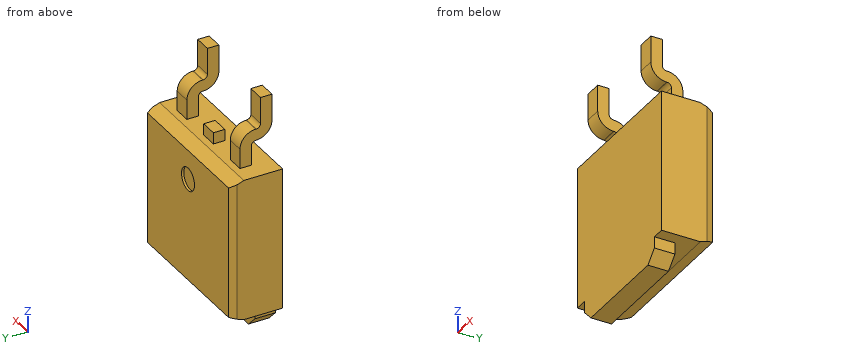
from build123d import *
from OCP.BRepFilletAPI import BRepFilletAPI_MakeChamfer

# Parameters (mm, degrees)
SKETCH1_W           = 6.5
SKETCH1_H           = 6.22
BOSS_EXTRUDE1_DEPTH = 2.3
SKETCH2_R           = 0.5
CUT_EXTRUDE1_DEPTH  = 0.1
SKETCH3_W           = 5.4
SKETCH3_H           = 0.9
BOSS_EXTRUDE2_DEPTH = 1
CHAMFER2_SIZE       = 0.5
SKETCH5_W           = 0.75
SKETCH5_H           = 0.5
SKETCH10_W          = 0.75
SKETCH10_H          = 0.5
BOSS_EXTRUDE3_DEPTH = 0.5
CHAMFER3_SIZE       = 0.6
CHAMFER3_SIZE2      = 0.218382141
CHAMFER4_SIZE       = 0.3
CHAMFER4_SIZE2      = 0.10919107


with BuildPart() as part:
    # Sketch1 → Boss-Extrude1 (new body)
    with BuildSketch(Plane(origin=(0, 0, 0), x_dir=(1, 0, 0), z_dir=(0, 1, 0))):
        with Locations((3.25, 3.11)):
            Rectangle(SKETCH1_W, SKETCH1_H)
    extrude(amount=BOSS_EXTRUDE1_DEPTH)

    # Sketch2 → Cut-Extrude1 (cut)
    with BuildSketch(Plane(origin=(0, 2.3, 0), x_dir=(1, 0, 0), z_dir=(0, 1, 0))):
        with Locations(Location((3.25, 1.5, 0), (0, 0, 270))):
            Circle(SKETCH2_R)
    extrude(amount=-CUT_EXTRUDE1_DEPTH, mode=Mode.SUBTRACT)

    # Sketch3 → Boss-Extrude2 (add)
    with BuildSketch(Plane(origin=(0, 0, -6.22), x_dir=(-1, 0, 0), z_dir=(0, 0, -1))):
        with Locations((-3.25, 0.45)):
            Rectangle(SKETCH3_W, SKETCH3_H)
    extrude(amount=BOSS_EXTRUDE2_DEPTH)

    # Chamfer2
    chamfer2_edges = [part.edges().sort_by_distance(p)[0] for p in [
        (5.95, 0.45, -7.22),
        (0.55, 0.45, -7.22),
    ]]
    chamfer(chamfer2_edges, length=CHAMFER2_SIZE)

    # Sweep2: sweep along a path in Sketch8
    with BuildLine(Plane(origin=(1.2, 0, 0), x_dir=(0, 0, -1), z_dir=(1, 0, 0))) as sweep2_path:
        Line((0, 1.15), (-0.860174932, 1.15))
        ThreePointArc((-0.860174932, 1.15), (-1.171301915, 1.021126984), (-1.300174932, 0.71))
        Line((-1.300174932, 0.71), (-1.300174932, 0.69))
        ThreePointArc((-1.300174932, 0.69), (-1.429047948, 0.378873016), (-1.740174932, 0.25))
        Line((-1.740174932, 0.25), (-2.900174932, 0.25))
    # Sketch5 → Sweep2 (sweep)
    with BuildSketch(Plane.XY):
        with Locations((1.2, 1.15)):
            Rectangle(SKETCH5_W, SKETCH5_H)
        with Locations((5.3, 1.15)):
            Rectangle(SKETCH5_W, SKETCH5_H)
    sweep(path=sweep2_path.line)

    # Sketch10 → Boss-Extrude3 (add)
    with BuildSketch(Plane.XY):
        with Locations((3.25, 1.15)):
            Rectangle(SKETCH10_W, SKETCH10_H)
    extrude(amount=BOSS_EXTRUDE3_DEPTH)

    # Chamfer3: one chamfer whose edges measure the first distance from different faces: ONE call of the kernel's chamfer builder (chamfer() names one face for all edges)
    chamfer3_edges_1 = [part.edges().sort_by_distance(p)[0] for p in [
        (3.25, 2.3, -6.22),
    ]]
    chamfer3_side_1 = [part.faces().sort_by_distance(p)[0] for p in [
        (3.25, 1.48716551, -6.22),
    ]]
    chamfer3_edges_2 = [part.edges().sort_by_distance(p)[0] for p in [
        (3.25, 2.3, 0),
    ]]
    chamfer3_side_2 = [part.faces().sort_by_distance(p)[0] for p in [
        (0.068949257, 1.15, 0),
    ]]
    chamfer3 = BRepFilletAPI_MakeChamfer(part.part.solid().wrapped)
    for e in chamfer3_edges_1:
        chamfer3.Add(CHAMFER3_SIZE, CHAMFER3_SIZE2, e.wrapped, chamfer3_side_1[0].wrapped)  # the first distance lies on this face
    for e in chamfer3_edges_2:
        chamfer3.Add(CHAMFER3_SIZE, CHAMFER3_SIZE2, e.wrapped, chamfer3_side_2[0].wrapped)  # the first distance lies on this face
    add(Compound.cast(chamfer3.Shape()), mode=Mode.REPLACE)

    # Chamfer4: one chamfer whose edges measure the first distance from different faces: ONE call of the kernel's chamfer builder (chamfer() names one face for all edges)
    chamfer4_edges_1 = [part.edges().sort_by_distance(p)[0] for p in [
        (0, 2.3, -3.11),
    ]]
    chamfer4_side_1 = [part.faces().sort_by_distance(p)[0] for p in [
        (0, 1.141218478, -3.11),
    ]]
    chamfer4_edges_2 = [part.edges().sort_by_distance(p)[0] for p in [
        (6.5, 2.3, -3.11),
    ]]
    chamfer4_side_2 = [part.faces().sort_by_distance(p)[0] for p in [
        (6.5, 1.141218478, -3.11),
    ]]
    chamfer4 = BRepFilletAPI_MakeChamfer(part.part.solid().wrapped)
    for e in chamfer4_edges_1:
        chamfer4.Add(CHAMFER4_SIZE, CHAMFER4_SIZE2, e.wrapped, chamfer4_side_1[0].wrapped)  # the first distance lies on this face
    for e in chamfer4_edges_2:
        chamfer4.Add(CHAMFER4_SIZE, CHAMFER4_SIZE2, e.wrapped, chamfer4_side_2[0].wrapped)  # the first distance lies on this face
    add(Compound.cast(chamfer4.Shape()), mode=Mode.REPLACE)


solid = part.part
Source: CAD feature listing. Evaluate the final solid. Frame: model axes, mm. Round coordinates to 2 decimals unless told otherwise and drop trailing zeros. Order: outer loops, then holes, each group sorted by start corner. A loop starts at its lowest first (then second) coordinate and runs counter-clockwise, first axis right, second up. Notation, with made-up numbers: (7, -30) - (53, -30) arc R26 ccw to (53, 3) - close; hole circle Ø9 at (-38, 16). An arc over 180 degrees is marked (long way). Use a Markdown table: item, result. Add a question column.
1. Section query C-C (y = 1). Return the cut outline in (x, z) (3 decimals).
2. First-contact query: pin 1 (0.8 mm diameter, centred on x = 1, z = 0.5, fed in from +Y); pin 2 (1.1 mm diameter, centred on x = 3.5, z = -1.5, fed in from +Y); pin 3 (0.7 mm diameter, centred on y = 0.5, z = 1.5, fed in from +X) (3 decimals); pin 4 (1.1 mm diameter, centred on y = 1, z = 2, fed in from -X) (3 decimals). Flat tips, straight axial feed; report the tip coordinate or a pass-through.
3. Section query D-D (z = -6.5). Return the cut outline in (x, y), then the cut area to 3 significant figures.
4. Line query: probe 1 along Z at (x, y) = (2.75, 0.6); probe 2 along X at (y, z) = (2.25, -1.5); probe 3 along Y at (x, z) = (5.25, 2.5). Output: solid intervals per line, ascending.
5. Section query B-B (x = 4). Return the cut outline in (y, z), then the cut area to 3 significant figures.
6. Section query A-A (y = 0.35). Return the cut outline in (x, z) (3 decimals).
Derived:
| question | item | result |
|---|---|---|
| 1 | outline | (0, -6.22) - (6.5, -6.22) - (6.5, 0) - (5.675, 0) - (5.675, 1.486) - (4.925, 1.486) - (4.925, 0) - (3.625, 0) - (3.625, 0.5) - (2.875, 0.5) - (2.875, 0) - (1.575, 0) - (1.575, 1.486) - (0.825, 1.486) - (0.825, 0) - (0, 0) - close |
| 2 | pin 1 | y = 1.4 |
| 2 | pin 2 | y = 2.3 |
| 2 | pin 3 | x = 5.675 |
| 2 | pin 4 | x = 0.825 |
| 3 | outline | (0.55, 0) - (5.95, 0) - (5.95, 0.9) - (0.55, 0.9) - close |
| 3 | area | 4.86 mm2 |
| 4 | probe 1 | -7.22 to 0 |
| 4 | probe 2 | 0.09 to 2.75, 3.75 to 6.41 |
| 4 | probe 3 | 0 to 0.5 |
| 5 | outline | (0, -7.22) - (0.9, -7.22) - (0.9, -6.22) - (1.7, -6.22) - (2.3, -6) - (2.3, -0.22) - (1.7, 0) - (0, 0) - close |
| 5 | area | 15.1 mm2 |
| 6 | outline | (0, -6.22) - (0.55, -6.22) - (0.55, -6.72) - (1.05, -7.22) - (5.45, -7.22) - (5.95, -6.72) - (5.95, -6.22) - (6.5, -6.22) - (6.5, 0) - (0, 0) - close; (0.825, 1.14) - (1.575, 1.14) - (1.575, 2.9) - (0.825, 2.9) - close; (4.925, 1.14) - (5.675, 1.14) - (5.675, 2.9) - (4.925, 2.9) - close |
